```python
from build123d import *

# Parameters (mm, degrees)
BOSS_EXTRUDE1_DEPTH = 6
SKETCH2_R           = 5.75
BOSS_EXTRUDE2_DEPTH = 12
FILLET1_R           = 0.5
SKETCH3_R           = 2
CUT_EXTRUDE1_DEPTH  = 19.0000001


with BuildPart() as part:
    # Sketch1 → Boss-Extrude1 (new body)
    with BuildSketch(Plane(origin=(0, 0, 0), x_dir=(1, 0, 0), z_dir=(0, 1, 0))):
        Polygon((1.209770832, 6.821763301), (-5.302934901, 4.458573924), (-6.512705733, -2.363189377), (-1.209770832, -6.821763301), (5.302934901, -4.458573924), (6.512705733, 2.363189377), align=None)
    extrude(amount=BOSS_EXTRUDE1_DEPTH)

    # Sketch2 → Boss-Extrude2 (add)
    with BuildSketch(Plane(origin=(0, 0, 0), x_dir=(-1, 0, 0), z_dir=(0, -1, 0))):
        Circle(SKETCH2_R)
    extrude(amount=BOSS_EXTRUDE2_DEPTH)

    # Fillet1
    fillet1_edges = [part.edges().sort_by_distance(p)[0] for p in [
        (5.75, 0, 0),
    ]]
    fillet(fillet1_edges, radius=FILLET1_R)

    # Sketch3 → Cut-Extrude1 (cut, through all)
    with BuildSketch(Plane(origin=(0, -12, 0), x_dir=(-1, 0, 0), z_dir=(0, -1, 0))):
        Circle(SKETCH3_R)
    extrude(amount=-CUT_EXTRUDE1_DEPTH, mode=Mode.SUBTRACT)


solid = part.part
```
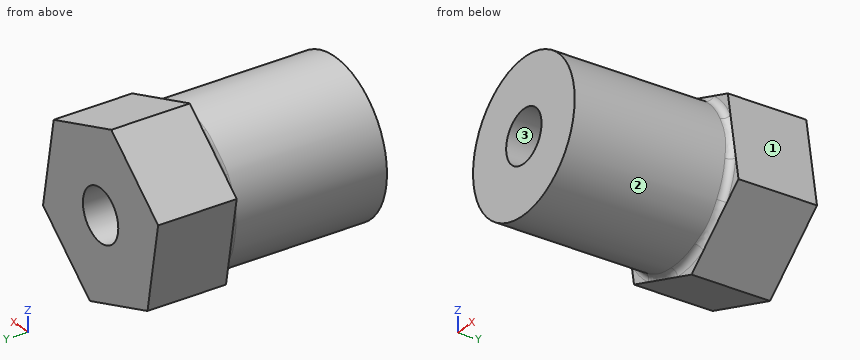
Geometry check sheet. Reference: the model listing, model coordinates, mm. Face numbers are marked on the shaded views. Coordinates: 2 decimals unless noted, no trailing zeros. Write each loop counter-clockwise with the first axis right and the second up, starting at its lowest first coordinate (ties: lowest second). Pieces come first, ordered by that corner, then holes. Notation, with made-up numbers: M 17,-17 L 53,-17 A8 cw 53,-6 Z; hole C 73,36.5 d1. An arc over 180 degrees is marked long. One line per item, written item: value. Start each with the question number.
(1) Scan lines: line 1 along Z through (x, y) = (0, -6); line 2 along Y through (x, z) = (-4.75, -4.25). Record each from-to range of solid material in increasing order. Write a range as [from, to].
(2) Depth check by flat-ended pin: pin 1 (3 mm diameter, centred on y = 0.5, z = -2, fed in from -X); pin 2 (5 mm diameter, centred on x = 0, z = 0, fed in from -Y); pin 3 (1 mm diameter, centred on x = 5, z = 4.5, fed in from -Y); pin 4 (4 mm diameter, centred on x = 3.5, y = -7.5, fed in from +Z). Enter the tip coordinate at first touch or a pass-through.
(3) Sectioned sample at A-A, the plane x = 0. Enter the section's corners in (y, z).
(4) Sectioned sample at C-C, the plane y = -1.25. Enter the section's corners in (x, z).
(5) Sectioned sample at B-B, the plane y = 4.5. Enter the section's corners in (x, z), and give its area (3 significant figures).
(6) Release check for a two-part mould opening along Z. For the marked faces 1, 2 and 3 record: released by +Z, released by -Z, zero draft, split by the parting line, or undercut.
Filled sheet:
1. line 1: [-5.75, -2], [2, 5.75]
1. line 2: [0, 6]
2. pin 1: x = -6
2. pin 2: y = -12
2. pin 3: y = 0
2. pin 4: z = 5.55
3. outline: M -12,-5.75 L -0.5,-5.75 A0.5 cw 0,-6.25 L 0,-6.38 L 6,-6.38 L 6,-2 L -12,-2 Z; M -12,2 L 6,2 L 6,6.38 L 0,6.38 L 0,6.25 A0.5 cw -0.5,5.75 L -12,5.75 Z
4. outline: C 0,0 d11.5; hole C 0,0 d4
5. outline: M -6.51,2.36 L -5.3,-4.46 L 1.21,-6.82 L 6.51,-2.36 L 5.3,4.46 L -1.21,6.82 Z; hole C 0,0 d4
5. area: 112 mm²
6. face 1: released by +Z
6. face 2: split by the parting line
6. face 3: undercut
